Read the model definition and answer for the solid it produces. Units are mm, in the model's axes. A direction names the side the tool comes from. Give positions to 0.01 mm unless a question says otherwise; leave off trailing zeros. Order: outer loops, then holes, each group sorted by start corner. A loop starts at its lowest first (then second) coordinate and runs counter-clockwise, first axis right, second up. Notation, with made-up numbers: (-27, -18) -> (3, -18) arc R15 ccw to (3, -5) -> close; hole circle Ø5 at (3, 40). An arc over 180 degrees is marked (long way). One line per question, with ' | ' between items. Start each with the question number.
```python
from build123d import *

# Parameters (mm, degrees)
BOSS_EXTRUDE1_DEPTH      = 127
BOSS_EXTRUDE5_REACH      = 249.033
BOSS_EXTRUDE5_END_RADIUS = 92.075
BOSS_EXTRUDE5_START      = -89.535
CUT_EXTRUDE4_REACH       = 159.498
CUT_EXTRUDE4_END_RADIUS  = 92.075
SKETCH9_W                = 12.7
SKETCH9_H                = 25.4


with BuildPart() as part:
    # Sketch1 → Boss-Extrude1 (new body)
    with BuildSketch(Plane(origin=(0, 0, 0), x_dir=(1, 0, 0), z_dir=(0, 1, 0))):
        with BuildLine():
            Line((-14.105106383, 90.988194833), (-13.716, 88.478175665))
            ThreePointArc((-13.716, 88.478175665), (-0.054221583, 89.534983582), (13.608826801, 88.494723335))
            Line((13.608826801, 88.494723335), (13.994892809, 91.00521194))
            ThreePointArc((13.994892809, 91.00521194), (-0.055759783, 92.074983116), (-14.105106383, 90.988194833))
        make_face()
    extrude(amount=BOSS_EXTRUDE1_DEPTH)

    # Boss-Extrude5: up to this cylinder (the profile starts inside it)
    boss_extrude5_end = Plane(origin=(0, -9.210463, 0), z_dir=(0, -1, 0)) * Cylinder(BOSS_EXTRUDE5_END_RADIUS, 683.216, mode=Mode.PRIVATE)
    # Sketch7 → Boss-Extrude5 (add, up to the surface)
    with BuildSketch(Plane.XY.offset(BOSS_EXTRUDE5_START), mode=Mode.PRIVATE) as boss_extrude5_sk1:
        with BuildLine():
            Line((-2.667, -16.51), (-2.667, 0))
            Line((-2.667, 0), (-7.493, 0))
            Line((-7.493, 0), (-7.493, -16.51))
            ThreePointArc((-7.493, -16.51), (-5.08, -18.923), (-2.667, -16.51))
        make_face()
    boss_extrude5_tool1 = extrude(boss_extrude5_sk1.sketch, amount=-BOSS_EXTRUDE5_REACH, mode=Mode.PRIVATE) & boss_extrude5_end
    add(boss_extrude5_tool1.solids().sort_by_distance((-5.08, -9.210463, -89.535))[0])
    # Sketch7 → Boss-Extrude5 (add, up to the surface)
    with BuildSketch(Plane.XY.offset(BOSS_EXTRUDE5_START), mode=Mode.PRIVATE) as boss_extrude5_sk2:
        with BuildLine():
            Line((2.667, 0), (2.667, -16.51))
            ThreePointArc((2.667, -16.51), (5.08, -18.923), (7.493, -16.51))
            Line((7.493, -16.51), (7.493, 0))
            Line((7.493, 0), (2.667, 0))
        make_face()
    boss_extrude5_tool2 = extrude(boss_extrude5_sk2.sketch, amount=-BOSS_EXTRUDE5_REACH, mode=Mode.PRIVATE) & boss_extrude5_end
    add(boss_extrude5_tool2.solids().sort_by_distance((5.08, -9.210463, -89.535))[0])

    # Cut-Extrude4: up to this cylinder (the profile starts inside it)
    cut_extrude4_end = Plane(origin=(0, 114.3, 0), z_dir=(0, -1, 0)) * Cylinder(CUT_EXTRUDE4_END_RADIUS, 504.146, mode=Mode.PRIVATE)
    # Sketch9 → Cut-Extrude4 (cut, up to the surface)
    with BuildSketch(Plane.XY, mode=Mode.PRIVATE) as cut_extrude4_sk1:
        with Locations((-0.389106383, 114.3)):
            Rectangle(SKETCH9_W, SKETCH9_H)
    cut_extrude4_tool1 = extrude(cut_extrude4_sk1.sketch, amount=-CUT_EXTRUDE4_REACH, mode=Mode.PRIVATE) & cut_extrude4_end
    add(cut_extrude4_tool1.solids().sort_by_distance((-0.389106, 114.3, 0))[0], mode=Mode.SUBTRACT)


solid = part.part
```
Q1. A cutting plane is placed at B-B, the plane z = -90.1. Determine the outline of the cut face in (x, y).
Q2. Determine the mould class of faces 4 (the flat face through (7.493, -8, -91)), 5 (the flat face through (-2.667, -8, -91)), 6 (the flat face through (10, 127, -90)) for opening direction X: pulls with the +X half, pulls with the -X half, needs draft (parallel to the pull), parting line crosses it, or undercut.
Q3. A cutting plane is placed at C-C, the plane y = 38. Determine the outline of the cut face in (x, z) (3 decimals), then the cut area to 3 significant figures.
Q4. Find the intervals of material crossed by line 1 (Y direction, x = -2.5, z = -91.35); line 2 (Y direction, x = 10.75, z = -89.2); line 3 (Z direction, x = 0, y = 30) (3 decimals), in increasing order.
Q5. Given P1, Ø0.7, axis at y = -4.5, z = -91, coming from the +X side; P2, Ø1.1, axis at x = 4, z = -90.5, coming from the -Y side; P3, Ø1.4, axis at x = -1.5, z = -90.5, coming from the +Y side; P4, Ø1.5, axis at x = -2.5, y = 103.5, coming from the -Z side, each flat-ended and moving along its own axis, determine where each tip first touches the part or whether it passes through.
Q6. Which of the six approach directions +Z, -Z, +X, -X, +Y, -Y give full straight-line access (tool end or side, diameter ignored) to faces 1 (the flat face through (-5, -9, -89.535)), 2 (the flat face through (-6.739, 114, -91)), 3 (the flat face through (2.667, -8, -91))?
Q7. A cutting plane is placed at D-D, the plane x = -5.08. Determine the outline of the cut face in (y, z) (3 decimals), then the cut area to 3 significant figures.
Q8. A cutting plane is placed at A-A, the plane y = 108. Determine the outline of the cut face in (x, z) (3 decimals), then the cut area to 3 significant figures.
Geometry results:
1) outline: (-13.97, 0) -> (-7.49, 0) -> (-7.49, -16.51) arc R2.41 ccw to (-2.67, -16.51) -> (-2.67, 0) -> (2.67, 0) -> (2.67, -16.51) arc R2.41 ccw to (7.49, -16.51) -> (7.49, 0) -> (13.86, 0) -> (13.86, 127) -> (5.96, 127) -> (5.96, 101.6) -> (-6.74, 101.6) -> (-6.74, 127) -> (-13.97, 127) -> close
2) face 4: pulls with the +X half | face 5: undercut | face 6: needs draft
3) outline: (-14.105, -90.988) arc R92.075 ccw to (13.995, -91.005) -> (13.609, -88.495) arc R89.535 cw to (-13.716, -88.478) -> close | area: 70.7 mm²
4) line 1: 0 to 101.6 | line 2: 0 to 127 | line 3: -92.075 to -89.535
5) P1: x = 7.49 | P2: y = -18.86 | P3: y = 101.6 | P4: through
6) face 1: +Z, +X, -X, -Y | face 2: +Z, -Z, +Y | face 3: +Z, -Z, -Y
7) outline: (-18.923, -91.935) -> (101.6, -91.935) -> (101.6, -89.391) -> (0, -89.391) -> (0, -89.535) -> (-18.923, -89.535) -> close | area: 304 mm²
8) outline: (-14.105, -90.988) arc R92.075 ccw to (-6.739, -91.828) -> (-6.739, -89.281) arc R89.535 cw to (-13.716, -88.478) -> close; (5.961, -91.882) arc R92.075 ccw to (13.995, -91.005) -> (13.609, -88.495) arc R89.535 cw to (5.961, -89.336) -> close | area: 38.4 mm²
